Read the model definition and answer for the solid it produces. Units are mm, in the model's axes. A direction names the side the tool comes from. Give positions to 0.01 mm unless a question says otherwise; leave off trailing zeros. Order: outer loops, then holes, each group sorted by start corner. A loop starts at its lowest first (then second) coordinate and runs counter-clockwise, first axis right, second up. Notation, with made-up numbers: (6, -18.75) - (31, -18.75) arc R27 cw to (31, -2.75) - close; hole circle Ø4 at (21, 38.5). An arc over 180 degrees is marked (long way). Write item = value, one per line.
```python
from build123d import *

# Parameters (mm, degrees)
F1_DEPTH  = 82
F2_W      = 52
F2_H      = 24
F3_DEPTH  = 15
F4_W      = 52
F4_H      = 24
F5_DEPTH  = 15
F6_R      = 9.75
F7_DEPTH  = 35.6
F8_R      = 6
F9_DEPTH  = 15.401
F10_R     = 3.25
F11_DEPTH = 20
F12_D     = 6.8
F12_DEPTH = 16
F12_TIP   = 2.0429261047


with BuildPart() as f1:
    # F0 (on Right) → F1 (new body)
    with BuildSketch(Plane.YZ):
        Polygon((0, 11), (0, 0), (82, 0), (82, 11), (67, 11), (67, 35), (82, 35), (82, 51), (0, 51), (0, 35), (15, 35), (15, 11), align=None)
    extrude(amount=F1_DEPTH)

    # F2 (on face) → F3 (cut)
    with BuildSketch(Plane.YZ.offset(82)):
        with Locations((41, 23)):
            Rectangle(F2_W, F2_H)
    extrude(amount=-F3_DEPTH, mode=Mode.SUBTRACT)

    # F4 (on face) → F5 (cut)
    with BuildSketch(Plane(origin=(0, 0, 0), x_dir=(0, -1, 0), z_dir=(-1, 0, 0))):
        with Locations((-41, 23)):
            Rectangle(F4_W, F4_H)
    extrude(amount=-F5_DEPTH, mode=Mode.SUBTRACT)

    # F6 (on face) → F7 (cut)
    with BuildSketch(Plane(origin=(0, 0, 0), x_dir=(1, 0, 0), z_dir=(0, 0, -1))):
        with Locations((41, -41)):
            Circle(F6_R)
    extrude(amount=-F7_DEPTH, mode=Mode.SUBTRACT)

    # F8 (on face) → F9 (cut, through all)
    with BuildSketch(Plane(origin=(0, 0, 35.6), x_dir=(1, 0, 0), z_dir=(0, 0, -1))):
        with Locations((41, -41)):
            Circle(F8_R)
    extrude(amount=-F9_DEPTH, mode=Mode.SUBTRACT)

    # F10 (on face) → F11 (cut)
    with BuildSketch(Plane.XY.offset(51)):
        with Locations((7.5, 7.5)):
            Circle(F10_R)
        with Locations((7.5, 29.8)):
            Circle(F10_R)
        with Locations((7.5, 52.1)):
            Circle(F10_R)
        with Locations((7.5, 74.4)):
            Circle(F10_R)
        with Locations((29.8, 7.5)):
            Circle(F10_R)
        with Locations((29.8, 74.4)):
            Circle(F10_R)
        with Locations((52.1, 7.5)):
            Circle(F10_R)
        with Locations((52.1, 74.4)):
            Circle(F10_R)
        with Locations((74.4, 7.5)):
            Circle(F10_R)
        with Locations((74.4, 29.8)):
            Circle(F10_R)
        with Locations((74.4, 52.1)):
            Circle(F10_R)
        with Locations((74.4, 74.4)):
            Circle(F10_R)
    extrude(amount=-F11_DEPTH, mode=Mode.SUBTRACT)

    # F12
    with Locations(Plane.XY.offset(51)):
        with Locations((7.5, 7.5), (7.5, 29.8), (7.5, 52.1), (7.5, 74.4), (29.8, 74.4), (52.1, 74.4), (74.4, 74.4), (74.4, 52.1), (74.4, 29.8), (74.4, 7.5), (52.1, 7.5), (29.8, 7.5)):
            Hole(F12_D / 2, depth=F12_DEPTH)
            with Locations((0, 0, -(F12_DEPTH + F12_TIP / 2))):  # 118° drill point
                Cone(0, F12_D / 2, F12_TIP, mode=Mode.SUBTRACT)


solid = f1.part
```
1. Determine the mould class of faces 1 (the face through (41, 15, 23)), 2 (the face through (13, 40, 35)), 3 (the face through (4.257, 30.821, 42.888)) for opening direction Y: +Y half, -Y half, draft (parallel to the pull), parting line (faces both ways), or undercut.
Recorded:
face_1 = -Y half
face_2 = draft
face_3 = undercut
2. Section A-A (y = 7.5) is taken. Determine the outline of the cut face in (x, z), and give its area (3 significant figures).
Recorded:
outline = (0, 0) - (82, 0) - (82, 11) - (0, 11) - close; (0, 35) - (4.1, 35) - (4.1, 51) - (0, 51) - close; (10.9, 35) - (26.4, 35) - (26.4, 51) - (10.9, 51) - close; (33.2, 35) - (48.7, 35) - (48.7, 51) - (33.2, 51) - close; (55.5, 35) - (71, 35) - (71, 51) - (55.5, 51) - close; (77.8, 35) - (82, 35) - (82, 51) - (77.8, 51) - close
area = 1,780 mm^2
3. Straight lines are drawn through the part: L1, parallel to Y at x = 7.5, z = 42.75; L2, parallel to X at y = 74, z = 42; L3, parallel to Z at x = 19, y = 71. For each, find the intervals that lie inside material, in ascending order. Write a range as [from, to].
Recorded:
L1 = [0, 4.1], [10.9, 26.4], [33.2, 48.7], [55.5, 71], [77.8, 82]
L2 = [0, 4.12], [10.88, 26.42], [33.18, 48.72], [55.48, 71.02], [77.78, 82]
L3 = [0, 11], [35, 51]
4. Section C-C (z = 8) is taken. Determine the outline of the cut face in (x, y).
Recorded:
outline = (0, 0) - (82, 0) - (82, 82) - (0, 82) - close; hole circle Ø19.5 at (41, 41)
5. Section D-D (y = 52.1) is taken. Determine the outline of the cut face in (x, z), and give its area (3 significant figures).
Recorded:
outline = (0, 0) - (82, 0) - (82, 11) - (67, 11) - (67, 35) - (71, 35) - (71, 51) - (10.9, 51) - (10.9, 35) - (15, 35) - (15, 11) - (0, 11) - close; (0, 35) - (4.1, 35) - (4.1, 51) - (0, 51) - close; (77.8, 35) - (82, 35) - (82, 51) - (77.8, 51) - close
area = 3,240 mm^2
6. For faces 4 (the face through (15, 41, 23)), 5 (the face through (71.157, 30.821, 42.888)), 6 (the face through (36.24, 44.65, 43.19)), 7 (the face through (38.89, 50.52, 17.55)), determine the directions among +Z, -Z, +X, -X, +Y, -Y from which every point of the face is accessible in a straight line to the end or side of a thin tool.
Recorded:
face_4 = -X, +Y, -Y
face_5 = +Z
face_6 = +Z, -Z
face_7 = -Z
7. Flat-ended cylindrical pins translate along their axes: pin 1 (4 mm diameter, centred on x = 74.4, y = 29.8, fed in from +Z); pin 2 (8 mm diameter, centred on x = 29.8, y = 74.4, fed in from -Z); pin 3 (5 mm diameter, centred on x = 49.5, z = 23.5, fed in from -Y); pin 4 (7 mm diameter, centred on y = 37.5, z = 21, fed in from -X). Find the tip coordinate at first contact, or state that the pin passes through.
Recorded:
pin_1 = 11
pin_2 = 0
pin_3 = 15
pin_4 = 15
